Check sheet for the drawn part. Datum: minimum x, y, z corner. Units: mm. A direction names the side the tool comes from. Coordinates: 2 decimals unless noted, no trailing zeros. Write each loop counter-clockwise with the first axis right and the second up, starting at its lowest first coordinate (ties: lowest second). Pieces come first, ordered by that corner, then holes. Notation, with made-up numbers: (-23.75, 41) - (28.25, 41) arc R20 ccw to (28.25, 63) - close; hole circle Ø4 at (89.25, -29.5). An arc over 180 degrees is marked (long way). Use CSV: the item, a comma, the result in double quotes. Start each with the question number.
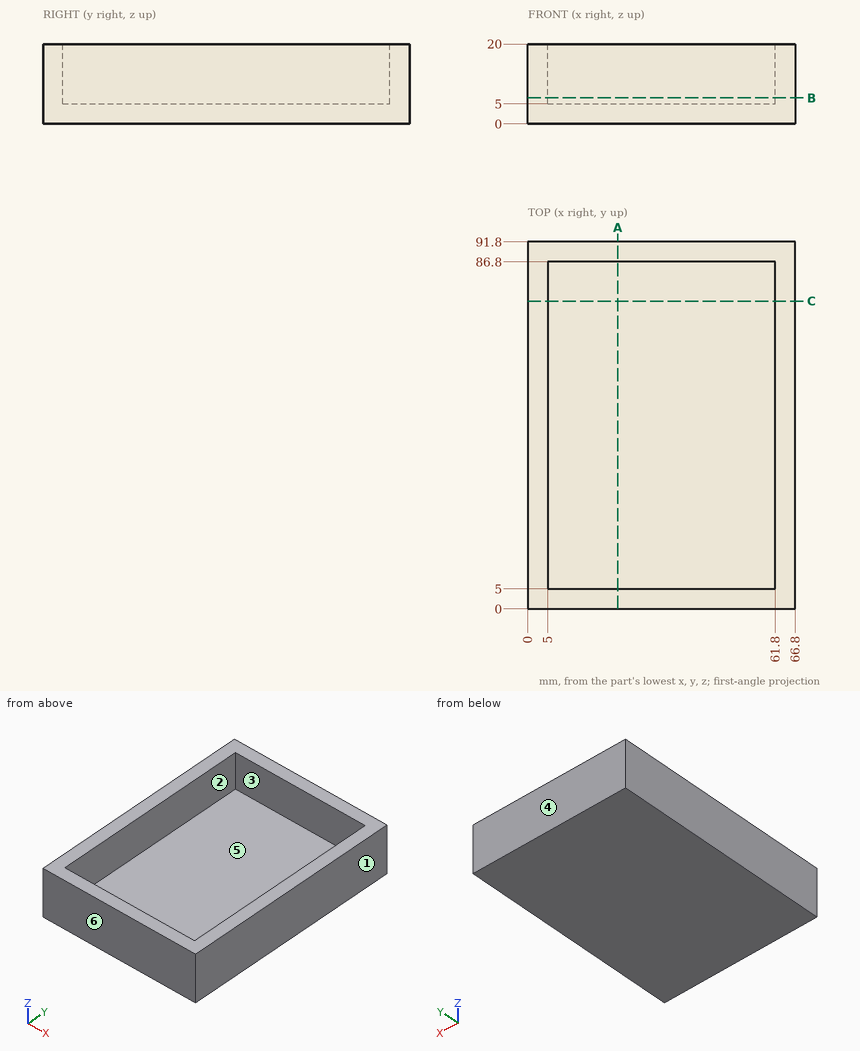
Q1. Gauge pin test, flat end, axial feed: pin 1 (17 mm diameter, centred on x = 37.5, y = 33, fed in from +Z). Record the tip position at first contact, or that the pin passes through.
Q2. Tool access check on the marked faces 5 and 6. Record the directions out of +Z, -Z, +X, -X, +Y, -Y that give a thin tool (end or side, any length) a straight path to the whole face; none if there is none.
Q3. Cross-section at A-A (x = 22.5). Record the cut outline in (y, z).
Q4. Scan lines: line 1 along Y through (x, z) = (37, 6); line 2 along X through (y, z) = (6, 5.75); line 3 along Z through (x, y) = (54.5, 15). Record each from-to range of solid material in increasing order. Write a range as from..to.
Q5. Cross-section at C-C (y = 77). Record the cut outline in (x, z), plus the area to 3 significant figures.
Q6. Release check for a two-part mould opening along X. For the marked faces 1, 2, 3 and 4 record: released by +X, released by -X, zero draft, split by the parting line, or undercut.
Q7. Cross-section at B-B (z = 6.5). Record the cut outline in (x, y).
Reply:
1,pin 1,"z = 5"
2,face 5,"+Z"
2,face 6,"+Z, -Z, +X, -X, -Y"
3,outline,"(0, 0) - (91.8, 0) - (91.8, 20) - (86.8, 20) - (86.8, 5) - (5, 5) - (5, 20) - (0, 20) - close"
4,line 1,"0..5, 86.8..91.8"
4,line 2,"0..5, 61.8..66.8"
4,line 3,"0..5"
5,outline,"(0, 0) - (66.8, 0) - (66.8, 20) - (61.8, 20) - (61.8, 5) - (5, 5) - (5, 20) - (0, 20) - close"
5,area,"484 mm^2"
6,face 1,"released by +X"
6,face 2,"undercut"
6,face 3,"undercut"
6,face 4,"zero draft"
7,outline,"(0, 0) - (66.8, 0) - (66.8, 91.8) - (0, 91.8) - close; hole (5, 5) - (61.8, 5) - (61.8, 86.8) - (5, 86.8) - close"
